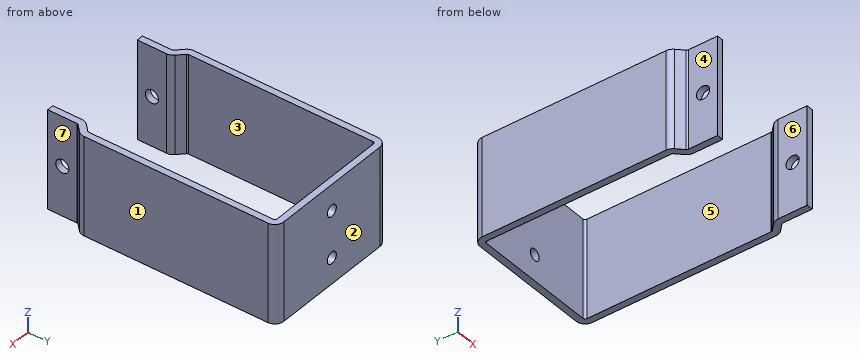
```python
from build123d import *

# Parameters (mm, degrees)
BASE_FLANGE1_DEPTH = 30
SKETCH9_R          = 2
CUT_EXTRUDE1_DEPTH = 84.600239234
SKETCH10_R         = 1.75
CUT_EXTRUDE2_DEPTH = 10


# Sheet-metal steps are written as plain solids
with BuildPart() as part:
    # Sketch1 → Base-Flange1 (new body)
    with BuildSketch(Plane.XY):
        with BuildLine():
            Line((-16.5, -5), (-16.5, 3.866463165))
            ThreePointArc((-16.5, 3.866463165), (-16.708311271, 4.913714646), (-17.301531583, 5.801531583))
            Line((-17.301531583, 5.801531583), (-19.284254855, 7.784254855))
            ThreePointArc((-19.284254855, 7.784254855), (-19.443929664, 8.023225094), (-19.5, 8.30510971))
            Line((-19.5, 8.30510971), (-19.5, 64.2634))
            ThreePointArc((-19.5, 64.2634), (-19.284254855, 64.784254855), (-18.7634, 65))
            Line((-18.7634, 65), (18.7634, 65))
            ThreePointArc((18.7634, 65), (19.284254855, 64.784254855), (19.5, 64.2634))
            Line((19.5, 64.2634), (19.5, 8.30510971))
            ThreePointArc((19.5, 8.30510971), (19.443929664, 8.023225094), (19.284254855, 7.784254855))
            Line((19.284254855, 7.784254855), (17.301531583, 5.801531583))
            ThreePointArc((17.301531583, 5.801531583), (16.708311271, 4.913714646), (16.5, 3.866463165))
            Line((16.5, 3.866463165), (16.5, -5))
            Line((16.5, -5), (18.5, -5))
            Line((18.5, -5), (18.5, 3.866463165))
            ThreePointArc((18.5, 3.866463165), (18.556070336, 4.148347781), (18.715745145, 4.38731802))
            Line((18.715745145, 4.38731802), (20.698468417, 6.370041293))
            ThreePointArc((20.698468417, 6.370041293), (21.291688729, 7.257858229), (21.5, 8.30510971))
            Line((21.5, 8.30510971), (21.5, 64.2634))
            ThreePointArc((21.5, 64.2634), (20.698468417, 66.198468417), (18.7634, 67))
            Line((18.7634, 67), (-18.7634, 67))
            ThreePointArc((-18.7634, 67), (-20.698468417, 66.198468417), (-21.5, 64.2634))
            Line((-21.5, 64.2634), (-21.5, 8.30510971))
            ThreePointArc((-21.5, 8.30510971), (-21.291688729, 7.257858229), (-20.698468417, 6.370041293))
            Line((-20.698468417, 6.370041293), (-18.715745145, 4.38731802))
            ThreePointArc((-18.715745145, 4.38731802), (-18.556070336, 4.148347781), (-18.5, 3.866463165))
            Line((-18.5, 3.866463165), (-18.5, -5))
            Line((-18.5, -5), (-16.5, -5))
        make_face()
    extrude(amount=BASE_FLANGE1_DEPTH)

    # Sketch9 → Cut-Extrude1 (cut, through all)
    with BuildSketch(Plane.ZY.offset(18.5)):
        with Locations((15, -0.566768417)):
            Circle(SKETCH9_R)
    extrude(amount=-CUT_EXTRUDE1_DEPTH, mode=Mode.SUBTRACT)

    # Sketch10 → Cut-Extrude2 (cut)
    with BuildSketch(Plane(origin=(0, 67, 0), x_dir=(1, 0, 0), z_dir=(0, 1, 0))):
        with Locations(Location((0, -22.108972385, 0), (0, 0, 270))):
            Circle(SKETCH10_R)
        with Locations(Location((0, -7.891027615, 0), (0, 0, 270))):
            Circle(SKETCH10_R)
    extrude(amount=-CUT_EXTRUDE2_DEPTH, mode=Mode.SUBTRACT)


solid = part.part
```
Input: part model. Units: mm. Frame: model coordinates. Face numbers are marked on the shaded views. A direction names the side the tool comes from. Coordinates: 2 decimals unless noted, no trailing zeros. Loops run counter-clockwise (first coordinate to the right, second up) from the corner with the lowest first, then second, coordinate; pieces in that order, holes last. Notation, with made-up numbers: (88.25, 21.5) - (104.25, 21.5) arc R20 ccw to (104.25, 28.5) - close; hole circle Ø1 at (-36, 28.25). An arc over 180 degrees is marked (long way). Answer in a Markdown table with one row per item.
(1) Cut plane A-A on y = 42.5. Output: boundary loops of the cut face in (x, z).
Model answer:
| item | result |
|---|---|
| outline | (-21.5, 0) - (-19.5, 0) - (-19.5, 30) - (-21.5, 30) - close; (19.5, 0) - (21.5, 0) - (21.5, 30) - (19.5, 30) - close |
(2) Pin query (flat end, axial travel): P1, Ø5, axis at y = -0.57, z = 15, coming from the +X side; P2, Ø1.5, axis at x = 3.5, z = 19.5, coming from the -Y side; P3, Ø2.5, axis at y = -2.5, z = 19.5, coming from the -X side. Return the tip coordinate at first contact, or that it passes through.
Model answer:
| item | result |
|---|---|
| P1 | stops at x = 18.5 |
| P2 | stops at y = 65 |
| P3 | stops at x = -18.5 |
(3) Cut plane C-C on z = 15. Count the separate pieces of the cut face and the enclosed holes in it, plus the area to 3 significant figures.
Model answer:
| item | result |
|---|---|
| separate pieces | 3 |
| enclosed holes | 0 |
| area | 351 mm² |
(4) Cut plane D-D on z = 2.5. Output: boundary loops of the cut face in (x, y).
Model answer:
| item | result |
|---|---|
| outline | (-21.5, 8.31) arc R2.74 ccw to (-20.7, 6.37) - (-18.72, 4.39) arc R0.74 cw to (-18.5, 3.87) - (-18.5, -5) - (-16.5, -5) - (-16.5, 3.87) arc R2.74 ccw to (-17.3, 5.8) - (-19.28, 7.78) arc R0.74 cw to (-19.5, 8.31) - (-19.5, 64.26) arc R0.74 cw to (-18.76, 65) - (18.76, 65) arc R0.74 cw to (19.5, 64.26) - (19.5, 8.31) arc R0.74 cw to (19.28, 7.78) - (17.3, 5.8) arc R2.74 ccw to (16.5, 3.87) - (16.5, -5) - (18.5, -5) - (18.5, 3.87) arc R0.74 cw to (18.72, 4.39) - (20.7, 6.37) arc R2.74 ccw to (21.5, 8.31) - (21.5, 64.26) arc R2.74 ccw to (18.76, 67) - (-18.76, 67) arc R2.74 ccw to (-21.5, 64.26) - close |
(5) Material intervals for L1, parallel to X at y = 22.5, z = 22; L2, parallel to X at y = 2.5, z = 18.5; L3, parallel to Y at x = -10, z = 17.5, sorted ascending. Write a range as from..to.
Model answer:
| item | result |
|---|---|
| L1 | x = -21.5..-19.5, 19.5..21.5 |
| L2 | x = -18.5..-16.5, 16.5..18.5 |
| L3 | y = 65..67 |
(6) Cut plane B-B on x = 0. Output: boundary loops of the cut face in (y, z), plus the area to 3 significant figures.
Model answer:
| item | result |
|---|---|
| outline | (65, 0) - (67, 0) - (67, 6.14) - (65, 6.14) - close; (65, 9.64) - (67, 9.64) - (67, 20.36) - (65, 20.36) - close; (65, 23.86) - (67, 23.86) - (67, 30) - (65, 30) - close |
| area | 46.0 mm² |
(7) Set-up query: the marked faces 4, 5, 6 and 7. Return all of +Z, -Z, +X, -X, +Y, -Y with unobstructed straight access to the full face (end or side cutting, diameter ignored); none if empty.
Model answer:
| item | result |
|---|---|
| face 4 | +Z, -Z, -X, -Y |
| face 5 | +Z, -Z |
| face 6 | +Z, -Z, -Y |
| face 7 | +Z, -Z, +X, -Y |
(8) Mould query, pull axis X, two halves, no side actions, for the marked faces 1, 2 and 3. Classes: pulls with the +X half, pulls with the -X half, needs draft (parallel to the pull), parting line crosses it, or undercut.
Model answer:
| item | result |
|---|---|
| face 1 | pulls with the +X half |
| face 2 | needs draft |
| face 3 | undercut |
